Verification items for the finished model (mm, model axes). A direction names the side the tool comes from. Give positions to 0.01 mm unless a question says otherwise; leave off trailing zeros. Order: outer loops, then holes, each group sorted by start corner. A loop starts at its lowest first (then second) coordinate and runs counter-clockwise, first axis right, second up.
from build123d import *

# Parameters (mm, degrees)
F0_R     = 27.0969905712
F1_DEPTH = 1.5
F2_R     = 5.028682338
F3_DEPTH = 2.5
F4_T     = -2.44
F5_DEPTH = 5


with BuildPart() as f1:
    # F0 (on Front) → F1 (new body, symmetric)
    with BuildSketch(Plane.XZ):
        Circle(F0_R)
    extrude(amount=F1_DEPTH, both=True)

    # F2 (on face) → F3 (join)
    with BuildSketch(Plane.XZ.offset(1.5)):
        Circle(F2_R)
    extrude(amount=F3_DEPTH)

    # F4
    f4_openings = [f1.faces().sort_by_distance(p)[0] for p in [
        (0, -4, 0),
    ]]
    offset(amount=F4_T, openings=f4_openings, kind=Kind.INTERSECTION)

    # F5 (add): a face of the model
    f5_faces = [f1.faces().sort_by_distance(p)[0] for p in [
        (0, -0.94, 0),
    ]]
    extrude(f5_faces, amount=F5_DEPTH)


solid = f1.part
(1) Go/stop test with flat-tipped pins: pin 1 (16.5 mm diameter, centred on x = 11, z = -2.5, fed in from -Y); pin 2 (2 mm diameter, centred on x = -12.5, y = -4, fed in from -Z); pin 3 (1.5 mm diameter, centred on x = 13.5, z = 11, fed in from -Y). Record where each tip stops, or that it passes through.
Solved:
pin 1: stops at y = -4
pin 2: passes through
pin 3: stops at y = -1.5
(2) Section check B-B, the plane x = 0. Enter the section's corners in (y, z).
Solved:
outline: (-5.94, -2.59) - (-4, -2.59) - (-4, -5.03) - (-1.5, -5.03) - (-1.5, -27.1) - (1.5, -27.1) - (1.5, 27.1) - (-1.5, 27.1) - (-1.5, 5.03) - (-4, 5.03) - (-4, 2.59) - (-5.94, 2.59) - close
(3) Section check C-C, the plane z = -15. Enter the section's corners in (x, y).
Solved:
outline: (-22.57, -1.5) - (22.57, -1.5) - (22.57, 1.5) - (-22.57, 1.5) - close
(4) Scan lines: line 1 (Y direction, x = -18, z = 1); line 2 (Z direction, x = -6.5, y = 0); line 3 (X direction, y = -0.5, z = 11.5). Record each from-to range of solid material in increasing order.
Solved:
line 1: y = -1.5 to 1.5
line 2: z = -26.31 to 26.31
line 3: x = -24.54 to 24.54
(5) Section check A-A, the plane z = 0. Enter the section's corners in (x, y), then the cut area to 3 significant figures.
Solved:
outline: (-27.1, -1.5) - (-5.03, -1.5) - (-5.03, -4) - (-2.59, -4) - (-2.59, -5.94) - (2.59, -5.94) - (2.59, -4) - (5.03, -4) - (5.03, -1.5) - (27.1, -1.5) - (27.1, 1.5) - (-27.1, 1.5) - close
area: 198 mm2
(6) Set-up check for faces 1 (the flat face through (2, -4, -2)), 2 (the flat face through (0, 1.5, 0)): record each of +Z, -Z, +X, -X, +Y, -Y from which the full face is reachable in a straight line by a thin tool's end or side.
Solved:
face 1: -Y
face 2: +Z, -Z, +X, -X, +Y
(7) Section check D-D, the plane x = 6. Enter the section's corners in (y, z).
Solved:
outline: (-1.5, -26.42) - (1.5, -26.42) - (1.5, 26.42) - (-1.5, 26.42) - close
